Can you work these out from the model? Positions are in its coordinate system, mm. A direction names the side the tool comes from. Round coordinates to 2 decimals unless told otherwise and drop trailing zeros. Loops run counter-clockwise (first coordinate to the right, second up) from the corner with the lowest first, then second, coordinate; pieces in that order, holes last. Notation, with made-up numbers: M 68,86 L 104,86 A20 ccw 104,106 Z; hole C 85,81.5 d7. An arc over 180 degrees is marked long. Return JSON: item names as keys, results as strings.
Autodesk Inventor part; units mm, degrees
ref_plane "YZ Plane" through (0, 0, 0) normal (1, 0, 0) x (0, 1, 0)
ref_plane "XZ Plane" through (0, 0, 0) normal (0, 1, 0) x (-1, 0, 0)
ref_plane "XY Plane" through (0, 0, 0) normal (0, 0, 1) x (1, 0, 0)
sketch "Sketch1" plane through (0, 0, 0) normal (0, 1, 0) x (-1, 0, 0)
  line L0 (0, 0) -> (102, 0)
  line L1 (102, 0) -> (102, -88)
  line L2 (102, -88) -> (0, -88)
  line L3 (0, -88) -> (0, 0)
  dimension "d0" = 102
  dimension "d1" = 88
extrude "Extrusion1" add sketch "Sketch1" along normal blind 10
shell "Shell1" thickness 1 removed faces 1 at (-68, 0, -29.3333)
sketch "Sketch2" plane through (-102, 0, 0) normal (0, 0, 1) x (1, 0, 0)
  line L0 (1, 0) -> (101, 0)
  line L1 (4.398, 0) -> (49.698, 0)
  line L2 (49.698, 0) -> (49.698, 3.6)
  line L3 (49.698, 3.6) -> (4.398, 3.6)
  line L4 (4.398, 3.6) -> (4.398, 0)
  line L5 (52.298, 0) -> (97.598, 0)
  line L6 (97.598, 0) -> (97.598, 3.6)
  line L7 (97.598, 3.6) -> (52.298, 3.6)
  line L8 (52.298, 3.6) -> (52.298, 0)
  line L9 (101, 0) -> (101, 9)
  point P0 (102, 0)
  point P1 (49.698, 0)
  dimension "d5" = 45.3
  dimension "d6" = 2.6
  dimension "d7" = 3.402
  dimension "d8" = 3.6
extrude "Extrusion2" cut sketch "Sketch2" against normal up to surface (1 mm away)
sketch "Sketch3" plane through (0, 0, 0) normal (1, 0, 0) x (0, 0, -1)
  line L0 (7.371, 0) -> (24.671, 0)
  line L1 (24.671, 0) -> (24.671, 3.6)
  line L2 (24.671, 3.6) -> (7.371, 3.6)
  line L3 (7.371, 3.6) -> (7.371, 0)
  line L4 (88, 0) -> (0, 0)
  line L5 (27.5, 0) -> (51.8, 0)
  line L6 (51.8, 0) -> (51.8, 3.6)
  line L7 (51.8, 3.6) -> (27.5, 3.6)
  line L8 (27.5, 3.6) -> (27.5, 0)
  line L9 (0, 3.6) -> (0, 0)
  line L10 (1, 0) -> (1, 9)
  dimension "d12" = 6.371
  dimension "d13" = 17.3
  dimension "d15" = 2.829
  dimension "d16" = 24.3
extrude "Extrusion3" cut sketch "Sketch3" against normal up to surface (1 mm away)
properties part number "TopCase"
Q1. Suppose I cut it at A-A, the plane y = 1.5. Please give me the cut outline in (x, z).
Results:
{"outline": "M -102,-88 L 0,-88 L 0,-51.8 L -1,-51.8 L -1,-87 L -101,-87 L -101,-1 L -97.6,-1 L -97.6,0 L -102,0 Z; M -52.3,-1 L -49.7,-1 L -49.7,0 L -52.3,0 Z; M -4.4,-1 L -1,-1 L -1,-7.37 L 0,-7.37 L 0,0 L -4.4,0 Z; M -1,-27.5 L 0,-27.5 L 0,-24.67 L -1,-24.67 Z"}
Q2. Suppose I cut it at B-B, the plane z = -26. Please give me the cut outline in (x, y), plus the area to 3 significant figures.
Results:
{"outline": "M -102,0 L -101,0 L -101,9 L -1,9 L -1,0 L 0,0 L 0,10 L -102,10 Z", "area": "120 mm2"}
Q3. Thinking about a two-plate mould opening in X: for faces 3 (the flat face through (-101, 4, -43)), 4 (the flat face through (-50, 6, 0)), 5 (the flat face through (-102, 5, -43)), which applies, pulls with the +X half, pulls with the -X half, needs draft (parallel to the pull), parting line crosses it, or undercut?
Results:
{"face 3": "undercut", "face 4": "needs draft", "face 5": "pulls with the -X half"}
Q4. Suppose I cut it at C-C, the plane x = -90. Please give me the cut outline in (y, z), plus the area to 3 significant figures.
Results:
{"outline": "M 0,-88 L 10,-88 L 10,0 L 3.6,0 L 3.6,-1 L 9,-1 L 9,-87 L 0,-87 Z", "area": "102 mm2"}
Q5. If I drill on line 1 along Z through (x, y) = (-39, 3.75); line 2 along X through (y, z) = (8, -26.5); line 3 along Y through (x, z) = (-50.5, -44.5), over which ranges is the centre line in solid material (lowest first)?
Results:
{"line 1": "z = -88 to -87, -1 to 0", "line 2": "x = -102 to -101, -1 to 0", "line 3": "y = 9 to 10"}
Q6. On a 3-axis mill with a long thin cutter (end or side, diameter ignored), from which of +Z, -Z, +X, -X, +Y, -Y can I reach the whole of each face in a straight line? I mean faces 1 (the flat face through (-52, 5, -88)), 2 (the flat face through (-50, 6, -1)). Say none if no direction works.
Results:
{"face 1": "-Z, +X, -X, +Y, -Y", "face 2": "-Y"}
Q7. I'm going to push flat-ended pins straight in: pin 1 Ø0.8 at (x, z) = (-0.5, -41.5) entering from -Y; pin 2 Ø2 at (x, z) = (-65.5, -54.5) entering from -Y; pin 3 Ø1.5 at (y, z) = (6, -58) entering from +X. Where does each tip first touch, or does it pass through?
Results:
{"pin 1": "stops at y = 3.6", "pin 2": "stops at y = 9", "pin 3": "stops at x = 0"}
